Design review of the part built by this model. Coordinates are the model's own, in mm. Face numbers are marked on the shaded views. A direction names the side the tool comes from. Coordinates: 2 decimals unless noted, no trailing zeros. Loops run counter-clockwise (first coordinate to the right, second up) from the corner with the lowest first, then second, coordinate; pieces in that order, holes last. Notation, with made-up numbers: M 24.5,-37.5 L 33.5,-37.5 A31 ccw 33.5,-0.5 Z; hole C 0,28 d6. An arc over 180 degrees is marked long. Answer as CSV lines item,"result". Start each with the question number.
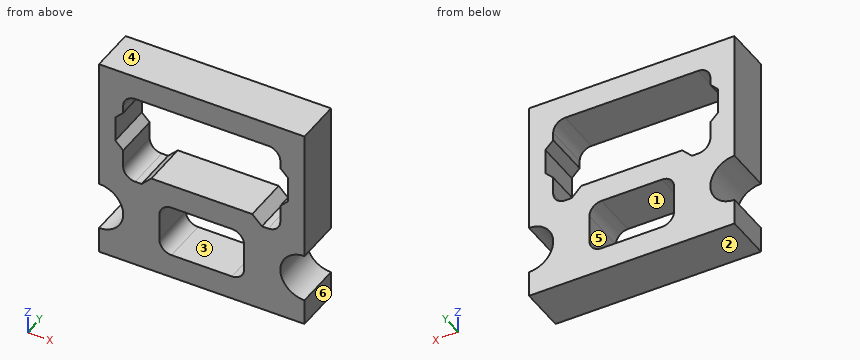
Autodesk Fusion 360 part; units mm, degrees
sketch "Sketch1" plane through (0, 0, 0) normal (0, 1, 0) x (1, 0, 0)
  line L0 (0, 0) -> (170, 0)
  line L1 (170, 0) -> (170, 170)
  line L2 (170, 170) -> (0, 170)
  line L3 (0, 170) -> (0, 0)
  line L4 (85, 170) -> (85, 128.5) construction
  line L5 (110, 107) -> (60, 107)
  line L6 (50, 117) -> (50, 140)
  line L7 (60, 150) -> (110, 150)
  line L8 (120, 140) -> (120, 117)
  line L9 (120, 107) -> (50, 150) construction
  line L10 (50, 107) -> (120, 150) construction
  arc A0 (60, 150) -> (50, 140) centre (60, 140) ccw
  arc A1 (120, 140) -> (110, 150) centre (110, 140) ccw
  arc A2 (110, 107) -> (120, 117) centre (110, 117) ccw
  arc A3 (50, 117) -> (60, 107) centre (60, 117) ccw
  line L11 (85, 128.5) -> (0, 128.5) construction
  line L12 (85, 128.5) -> (170, 128.5) construction
  arc A4 (0, 108.5) -> (0, 148.5) centre (0, 128.5) ccw
  arc A5 (170, 148.5) -> (170, 108.5) centre (170, 128.5) ccw
  line L13 (85, 0) -> (85, 53.5) construction
  line L14 (140, 20) -> (30, 20)
  line L15 (20, 30) -> (20, 87)
  line L16 (150, 87) -> (150, 30)
  line L17 (150, 20) -> (20, 87) construction
  line L18 (20, 20) -> (150, 87) construction
  arc A6 (20, 30) -> (30, 20) centre (30, 30) ccw
  arc A7 (140, 20) -> (150, 30) centre (140, 30) ccw
  line L19 (85, 53.5) -> (20, 53.5) construction
  line L20 (85, 53.5) -> (150, 53.5) construction
  line L21 (20, 53.5) -> (13.5, 53.5) construction
  line L22 (13.5, 53.5) -> (13.5, 64)
  line L23 (13.5, 53.5) -> (13.5, 43)
  line L24 (13.5, 43) -> (13.5, 36.5) construction
  line L25 (13.5, 36.5) -> (20, 36.5) construction
  line L26 (13.5, 64) -> (13.5, 70.5) construction
  line L27 (13.5, 70.5) -> (20, 70.5) construction
  line L28 (13.5, 64) -> (20, 70.5)
  line L29 (13.5, 43) -> (20, 36.5)
  line L30 (156.5, 64) -> (150, 70.5)
  line L31 (156.5, 53.5) -> (156.5, 64)
  line L32 (156.5, 53.5) -> (156.5, 43)
  line L33 (156.5, 43) -> (150, 36.5)
  line L34 (85, 53.5) -> (85, 87) construction
  line L35 (85, 128.5) -> (85, 87) construction
  line L36 (85, 87) -> (43.25, 87)
  line L37 (43.25, 87) -> (35.25, 95)
  line L38 (30, 95) -> (35.25, 95)
  line L39 (35.25, 95) -> (35.25, 87) construction
  line L40 (35.25, 87) -> (43.25, 87) construction
  line L41 (30, 95) -> (30, 85) construction
  arc A8 (30, 95) -> (20, 85) centre (30, 85) ccw
  line L42 (30, 85) -> (30, 95) construction
  line L43 (30, 85) -> (20, 85) construction
  arc A9 (150, 85) -> (140, 95) centre (140, 85) ccw
  line L44 (140, 95) -> (134.75, 95)
  line L45 (126.75, 87) -> (134.75, 95)
  line L46 (85, 87) -> (126.75, 87)
  point P0 (85, 128.5)
  point P1 (85, 53.5)
  dimension "d1" = 170
  dimension "d2" = 170
  dimension "d19" = 41.5
  dimension "d20" = 70
  dimension "d21" = 43
  dimension "d22" = 10
  dimension "d23" = 10
  dimension "d24" = 10
  dimension "d25" = 10
  dimension "d26" = 20
  dimension "d27" = 20
  dimension "d28" = 53.5
  dimension "d29" = 130
  dimension "d30" = 67
  dimension "d31" = 10
  dimension "d32" = 10
  dimension "d33" = 6.5
  dimension "d34" = 10.5
  dimension "d35" = 10.5
  dimension "d36" = 6.5
  dimension "d37" = 6.5
  dimension "d41" = 41.5
  dimension "d42" = 33.5
  dimension "d44" = 41.75
  dimension "d48" = 5.25
  dimension "d49" = 135
  dimension "d50" = 8
  dimension "d51" = 10
  dimension "d52" = 90
  dimension "d53" = 135
  dimension "d54" = 8
extrude "Extrude1" add sketch "Sketch1" along normal blind 38.1 contours L0 L1 L2 L3 A4 A5
Item 1: Add section C-C (x = 90.5). Give the boundary of the cut face in (y, z), plus the area to 3 significant figures.
Item 2: Add section D-D (y = 17). Give the number of separate pieces and of enclosed holes in the cut face, plus the area to 3 significant figures.
Item 3: Mouldability with a two-part tool opening along Z and no side actions: class the marked faces 1, 2, 3 and 4 as released by +Z, released by -Z, zero draft, split by the parting line, or undercut.
Item 4: For the marked faces 5 and 6, list the 3-axis set-ups (+Z, -Z, +X, -X, +Y, -Y) from which the entire face can be reached by the end or side of a thin tool; tool diameter is ignored.
Item 5: Add section A-A (x = 32.5). Give the boundary of the cut face in (y, z).
Item 6: For pin 1 (4 mm diameter, centred on y = 31.5, z = -144.5, fed in from -X); pin 2 (7 mm diameter, centred on y = 16, z = -127, fed in from -X), all flat-tipped, find the tip position at first contact; note any pin that passes through.
Item 7: For line 1 along Z through (x, y) = (80.5, 32); line 2 along Z through (x, y) = (125, 26); line 3 along Z through (x, y) = (135, 28.5), list the stretches that pass through material, from the lowest coordinate up. Write a range as from..to.
Item 8: Add section B-B (z = -128.5). Give the boundary of the cut face in (x, y), plus the area to 3 significant figures.
Response:
1,outline,"M 0,-170 L 38.1,-170 L 38.1,-150 L 0,-150 Z; M 0,-107 L 38.1,-107 L 38.1,-87 L 0,-87 Z; M 0,-20 L 38.1,-20 L 38.1,0 L 0,0 Z"
1,area,"2,290 mm²"
2,separate pieces,"1"
2,enclosed holes,"2"
2,area,"15,400 mm²"
3,face 1,"undercut"
3,face 2,"released by -Z"
3,face 3,"undercut"
3,face 4,"released by +Z"
4,face 5,"+Y, -Y"
4,face 6,"+Z, -Z, +X, +Y, -Y"
5,outline,"M 0,-170 L 38.1,-170 L 38.1,-95 L 0,-95 Z; M 0,-20 L 38.1,-20 L 38.1,0 L 0,0 Z"
6,pin 1,"x = 8.72"
6,pin 2,"x = 19.36"
7,line 1,"-170..-150, -107..-87, -20..0"
7,line 2,"-170..-87, -20..0"
7,line 3,"-170..-95, -20..0"
8,outline,"M 20,0 L 50,0 L 50,38.1 L 20,38.1 Z; M 120,0 L 150,0 L 150,38.1 L 120,38.1 Z"
8,area,"2,290 mm²"
